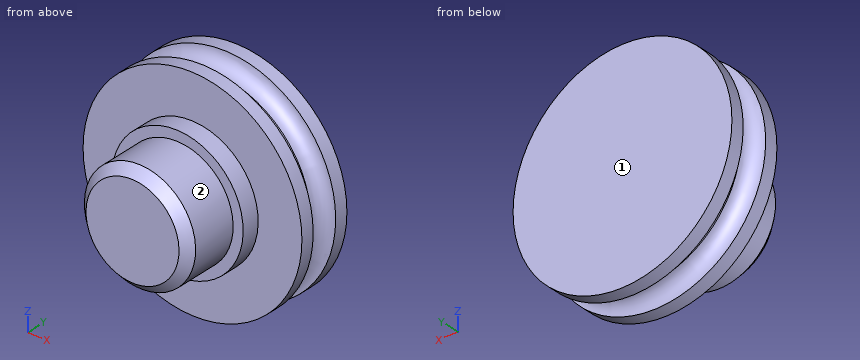
from build123d import *

# Parameters (mm, degrees)
SKETCH1_R           = 3.05
BOSS_EXTRUDE1_DEPTH = 3
SKETCH4_R           = 3.6
BOSS_EXTRUDE3_DEPTH = 1
SKETCH2_R           = 6
BOSS_EXTRUDE2_DEPTH = 3
SKETCH3_R           = 0.75
CHAMFER1_SIZE       = 0.5


with BuildPart() as part:
    # Sketch1 → Boss-Extrude1 (new body)
    with BuildSketch(Plane(origin=(0, 0, 0), x_dir=(1, 0, 0), z_dir=(0, 1, 0))):
        with Locations(Location((0, 0, 0), (0, 0, 270))):
            Circle(SKETCH1_R)
    extrude(amount=BOSS_EXTRUDE1_DEPTH)

    # Sketch4 → Boss-Extrude3 (add)
    with BuildSketch(Plane(origin=(0, 3, 0), x_dir=(1, 0, 0), z_dir=(0, 1, 0))):
        with Locations(Location((0, 0, 0), (0, 0, 270))):
            Circle(SKETCH4_R)
    extrude(amount=BOSS_EXTRUDE3_DEPTH)

    # Sketch2 → Boss-Extrude2 (add)
    with BuildSketch(Plane(origin=(0, 4, 0), x_dir=(1, 0, 0), z_dir=(0, 1, 0))):
        with Locations(Location((0, 0, 0), (0, 0, 270))):
            Circle(SKETCH2_R)
    extrude(amount=BOSS_EXTRUDE2_DEPTH)

    # Sketch3 → Cut-Revolve1 (revolve, cut)
    with BuildSketch(Plane.XY, mode=Mode.PRIVATE) as cut_revolve1_sk:
        with Locations((-6, 5.5)):
            Circle(SKETCH3_R)
    revolve(cut_revolve1_sk.sketch.rotate(Axis((0, 9.115200414, 0), (0, -1, 0)), 270), axis=Axis((0, 9.115200414, 0), (0, -1, 0)), mode=Mode.SUBTRACT)

    # Chamfer1
    chamfer1_edges = [part.edges().sort_by_distance(p)[0] for p in [
        (0, 0, -3.05),
    ]]
    chamfer(chamfer1_edges, length=CHAMFER1_SIZE)


solid = part.part
Work out the finished part from the listing and answer in its coordinate system (mm). Face numbers are marked on the shaded views. A direction names the side the tool comes from. Round coordinates to 2 decimals unless told otherwise and drop trailing zeros. Loops run counter-clockwise (first coordinate to the right, second up) from the corner with the lowest first, then second, coordinate; pieces in that order, holes last. Notation, with made-up numbers: (-13.75, 67) -> (10.25, 67) arc R19 cw to (10.25, 100) -> close; hole circle Ø4 at (19, 25). An arc over 180 degrees is marked (long way). Use one line per item in the form item = value.
(1) Find section D-D on y = 1. Give the vertices of the cut face in (x, z).
Answer list:
outline = circle Ø6.1 at (0, 0)
(2) Find section A-A on z = 0. Give the vertices of the cut face in (x, y), then the cut area to 3 significant figures.
Answer list:
outline = (-6, 4) -> (-3.6, 4) -> (-3.6, 3) -> (-3.05, 3) -> (-3.05, 0.5) -> (-2.55, 0) -> (2.55, 0) -> (3.05, 0.5) -> (3.05, 3) -> (3.6, 3) -> (3.6, 4) -> (6, 4) -> (6, 4.75) arc R0.75 cw to (6, 6.25) -> (6, 7) -> (-6, 7) -> (-6, 6.25) arc R0.75 cw to (-6, 4.75) -> close
area = 59.5 mm2
(3) Find section C-C on y = 3.25. Give the vertices of the cut face in (x, z), then the cut area to 3 significant figures.
Answer list:
outline = circle Ø7.2 at (0, 0)
area = 40.7 mm2
(4) Flat-ended cylindrical pins translate along their axes: P1, Ø4, axis at y = 3, z = -2, coming from the -X side; P2, Ø1, axis at y = 1, z = -3, coming from the -X side. Find the tip coordinate at first contact, or state that the pin passes through.
Answer list:
P1 = -5.99
P2 = -1.75
(5) Straight lines are drawn through the part: line 1 (Y direction, x = -3.75, z = 2.5); line 2 (Y direction, x = -3.5, z = -4.5); line 3 (Y direction, x = -1.5, z = 2.75). For each, find the intervals that lie inside material, in ascending order.
Answer list:
line_1 = 4 to 7
line_2 = 4 to 4.81, 6.19 to 7
line_3 = 3 to 7
(6) Find section B-B on x = 0. Give the vertices of the cut face in (y, z), then the cut area to 3 significant figures.
Answer list:
outline = (0, -2.55) -> (0.5, -3.05) -> (3, -3.05) -> (3, -3.6) -> (4, -3.6) -> (4, -6) -> (4.75, -6) arc R0.75 cw to (6.25, -6) -> (7, -6) -> (7, 6) -> (6.25, 6) arc R0.75 cw to (4.75, 6) -> (4, 6) -> (4, 3.6) -> (3, 3.6) -> (3, 3.05) -> (0.5, 3.05) -> (0, 2.55) -> close
area = 59.5 mm2
(7) A tool of negligible diameter and unlimited length cuts with its end or side. For the marked faces 1 and 2, from which of +Z, -Z, +X, -X, +Y, -Y can it reach the whole face along a straight path? Write none if from no direction.
Answer list:
face_1 = +Z, -Z, +X, -X, +Y
face_2 = -Y
